Could you check a few things on this drawing? It's one solid part, dimensions in mm from its lowest x, y, z. A direction names the side the tool comes from. Give positions to 0.01 mm unless a question says otherwise; leave off trailing zeros. Order: outer loops, then holes, each group sorted by start corner. A loop starts at its lowest first (then second) coordinate and runs counter-clockwise, first axis right, second up.
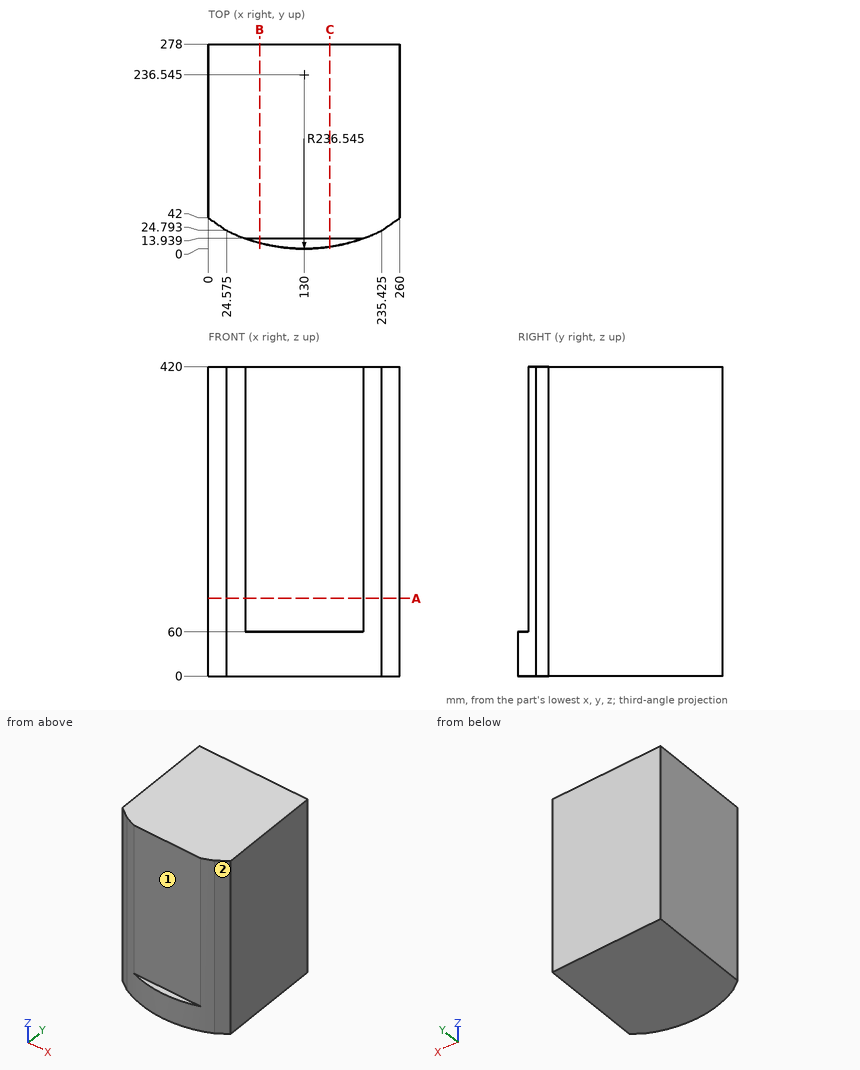
Q1. I'm going to push flat-ended pins straight in: P1, Ø2, axis at x = 78.5, y = 50, coming from the -Z side; P2, Ø2, axis at x = 171, z = 202.5, coming from the -Y side; P3, Ø7, axis at x = 112.5, y = 8.5, coming from the +Z side. Where does each tip first touch, or does it pass through?
Filled sheet:
P1: stops at z = 0
P2: stops at y = 13.94
P3: stops at z = 60
Q2. If we section it at B-B on x = 69.5: List the corners of the cut face in (y, z) for me.
Filled sheet:
outline: (7.87, 0) - (278, 0) - (278, 420) - (13.94, 420) - (13.94, 60) - (7.87, 60) - close
Q3. If we section it at A-A on z = 105.5: List the corners of the cut face in (x, y) for me (1 decimal).
Filled sheet:
outline: (0, 42) - (24.6, 24.8) arc R236.5 ccw to (50, 13.9) - (210, 13.9) arc R236.5 ccw to (235.4, 24.8) - (260, 42) - (260, 278) - (0, 278) - close
Q4. I need wall thicknesses on L1, parallel to Y at x = 106, z = 285; L2, parallel to Y at x = 230, z = 46. Which ranges of each line are inside material? Lowest first, please.
Filled sheet:
L1: y = 13.94 to 278
L2: y = 22.18 to 278
Q5. For the marked faces 1 and 2, which set-ups out of +Z, -Z, +X, -X, +Y, -Y let a thin tool reach every point of the face, with its end or its side?
Filled sheet:
face 1: +Z, +X, -X, -Y
face 2: +Z, -Z, +X, -Y
Q6. If we section it at C-C on x = 165: List the corners of the cut face in (y, z) for me, plus the area to 3 significant figures.
Filled sheet:
outline: (2.6, 0) - (278, 0) - (278, 420) - (13.94, 420) - (13.94, 60) - (2.6, 60) - close
area: 112,000 mm2
